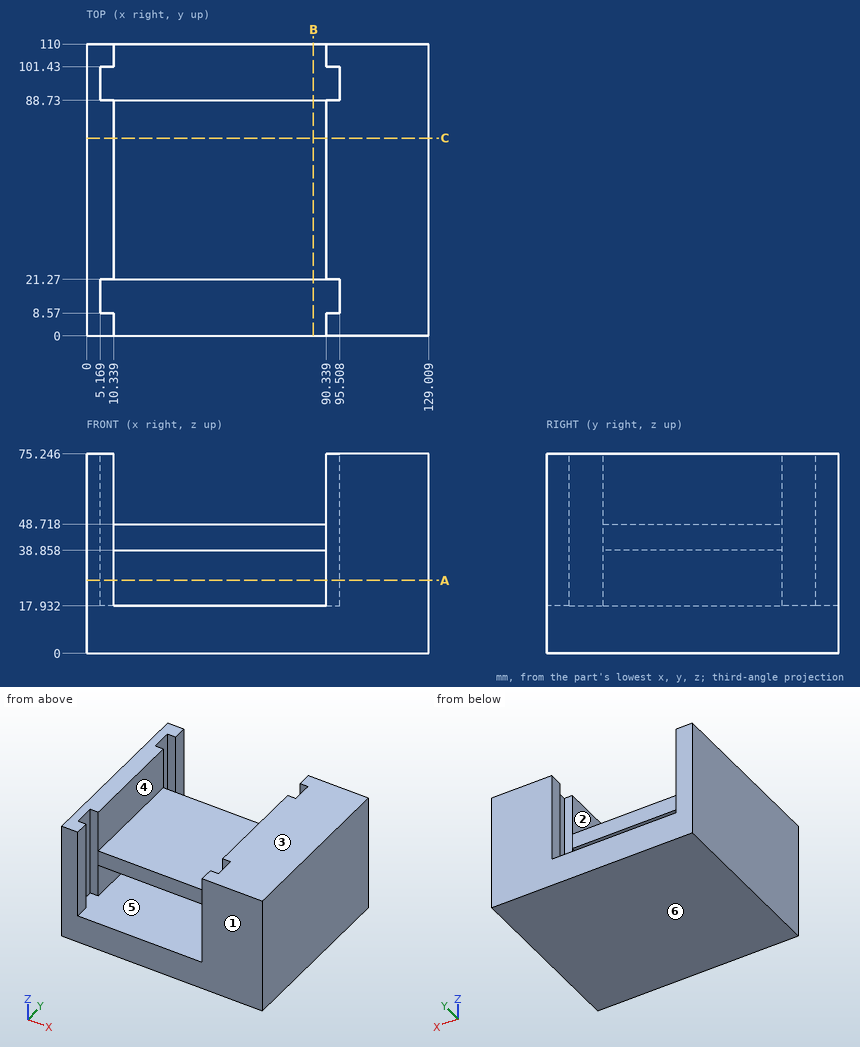
Part print with two shaded views. Sizes in mm from the minimum x, y, z corner. A direction names the side the tool comes from. Round coordinates to 2 decimals unless told otherwise and drop trailing zeros. Order: outer loops, then holes, each group sorted by start corner. A loop starts at its lowest first (then second) coordinate and runs counter-clockwise, first axis right, second up. Notation, with made-up numbers: M 79,85 L 103,85 A26 cw 103,113 Z; hole C -31,62.5 d1. An arc over 180 degrees is marked long. Put each result on its own line as item: value. Start each with the question number.
1. Tool access for the marked faces 1 and 2: list every direction of +Z, -Z, +X, -X, +Y, -Y with a clear straight run to the whole face (end or side of a thin tool).
2. Drop flat-ended pins along their axis: pin 1 (2.5 mm diameter, centred on x = 7.5, z = 50, fed in from -Y); pin 2 (5 mm diameter, centred on x = 67.5, z = 42.5, fed in from +Y). Give the stop position or say it passes through.
3. Drill centre lines: probe 1 along Y at (x, z) = (92, 18.5); probe 2 along Z at (x, y) = (24.5, 47); probe 3 along X at (y, z) = (54, 31.5). Where is each one in solid material? Low to high. Write a range as [from, to].
4. Slice it at A-A on z = 27.5. List the corners of the cut face in (x, y).
5. Slice it at B-B on x = 85.5. List the corners of the cut face in (y, z).
6. Slice it at C-C on y = 74.5. List the corners of the cut face in (x, z) (1 decimal).
7. Two-plate mould, pull along Z, no slides. Class the marked faces 3, 4, 5 and 6: +Z half, -Z half, draft (parallel to the pull), parting line (faces both ways), or undercut.
Findings:
1. face 1: +Z, -Z, +X, -X, -Y
1. face 2: +Z, +Y, -Y
2. pin 1: y = 0
2. pin 2: y = 88.73
3. probe 1: [0, 8.57], [21.27, 88.73], [101.43, 110]
3. probe 2: [0, 17.93], [38.86, 48.72]
3. probe 3: [0, 10.34], [90.34, 129.01]
4. outline: M 0,0 L 10.34,0 L 10.34,8.57 L 5.17,8.57 L 5.17,21.27 L 10.34,21.27 L 10.34,88.73 L 5.17,88.73 L 5.17,101.43 L 10.34,101.43 L 10.34,110 L 0,110 Z; M 90.34,0 L 129.01,0 L 129.01,110 L 90.34,110 L 90.34,101.43 L 95.51,101.43 L 95.51,88.73 L 90.34,88.73 L 90.34,21.27 L 95.51,21.27 L 95.51,8.57 L 90.34,8.57 Z
5. outline: M 0,0 L 110,0 L 110,17.93 L 0,17.93 Z; M 21.27,38.86 L 88.73,38.86 L 88.73,48.72 L 21.27,48.72 Z
6. outline: M 0,0 L 129,0 L 129,75.2 L 90.3,75.2 L 90.3,48.7 L 10.3,48.7 L 10.3,75.2 L 0,75.2 Z; hole M 10.3,17.9 L 90.3,17.9 L 90.3,38.9 L 10.3,38.9 Z
7. face 3: +Z half
7. face 4: draft
7. face 5: undercut
7. face 6: -Z half
